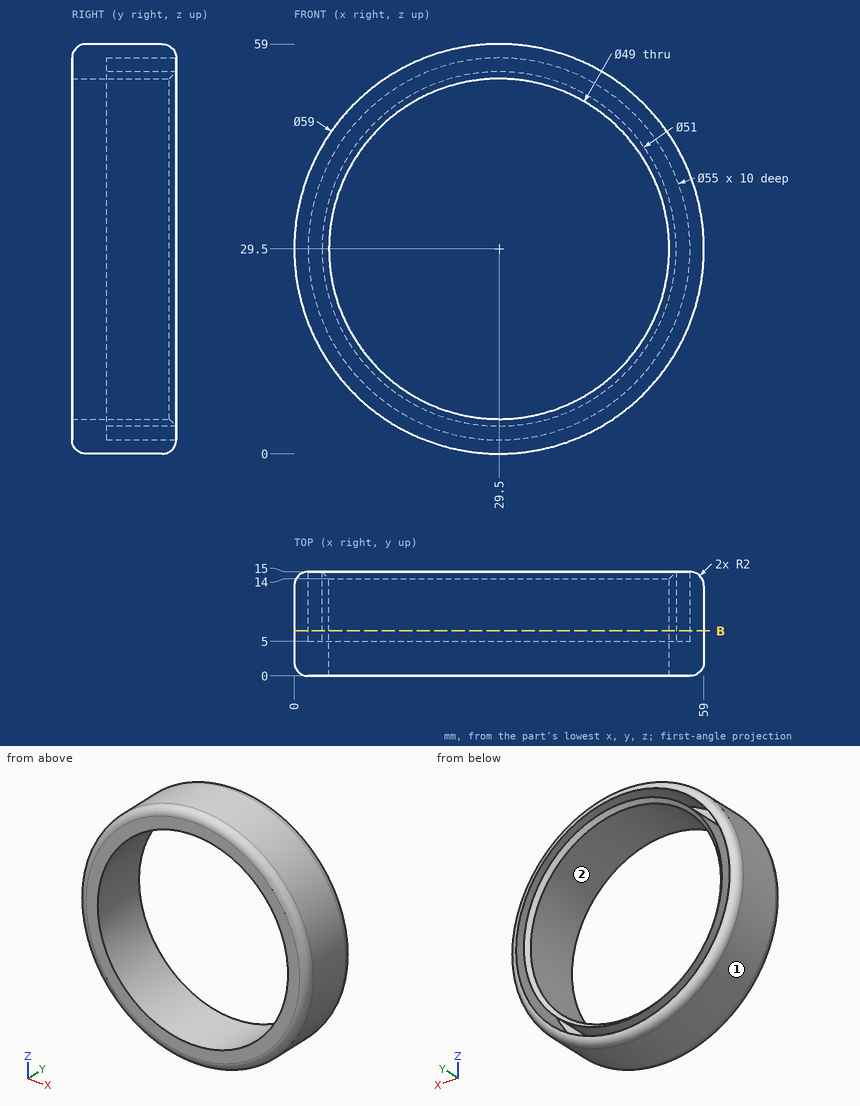
Input: dimensioned drawing with shaded views. Units: mm. Origin: part minimum x, y, z. Coordinates: 2 decimals unless noted, no trailing zeros. Loops run counter-clockwise (first coordinate to the right, second up) from the corner with the lowest first, then second, coordinate; pieces in that order, holes last.
Q1. Section B-B, the plane y = 6.5. Return the cut outline in (x, z), and give its area (3 significant figures).
Results are:
outline: circle Ø59 at (29.5, 29.5); circle Ø51 at (29.5, 29.5); hole circle Ø55 at (29.5, 29.5); hole circle Ø49 at (29.5, 29.5)
area: 515 mm2
Q2. Mould query, pull axis X, two halves, no side actions, for the marked faces 1 and 2. Classes: +X half, -X half, draft (parallel to the pull), parting line (faces both ways), or undercut.
Results are:
face 1: parting line
face 2: undercut
Q3. Line query: line 1 along Z through (x, y) = (29.5, 7.25); line 2 along Z through (x, y) = (23.5, 5.25); line 3 along X through (y, z) = (12.5, 20). Output: solid intervals per line, ascending.
Results are:
line 1: z = 0 to 2, 4 to 5, 54 to 55, 57 to 59
line 2: z = 0.62 to 2.66, 4.72 to 5.75, 53.25 to 54.28, 56.34 to 58.38
line 3: x = 1.57 to 3.69, 5.84 to 6.92, 52.08 to 53.16, 55.31 to 57.43
Q4. Contact query for flat-ended pins moving along their axis: pin 1 (3 mm diameter, centred on x = 28, y = 12, fed in from -Z); pin 2 (1 mm diameter, centred on y = 8, z = 12, fed in from +X); pin 3 (10 mm diameter, centred on x = 32.5, z = 48.5, fed in from -Y); pin 4 (8 mm diameter, centred on y = 9.5, z = 7, fed in from +X). Output: stop coordinate, or through.
Results are:
pin 1: stops at z = 0
pin 2: stops at x = 53.61
pin 3: passes through
pin 4: stops at x = 52.48
